Check sheet for the drawn part. Datum: minimum x, y, z corner. Units: mm. A direction names the side the tool comes from. Give positions to 0.01 mm unless a question says otherwise; leave off trailing zeros. Order: outer loops, then holes, each group sorted by start corner. A loop starts at its lowest first (then second) coordinate and runs counter-clockwise, first axis right, second up.
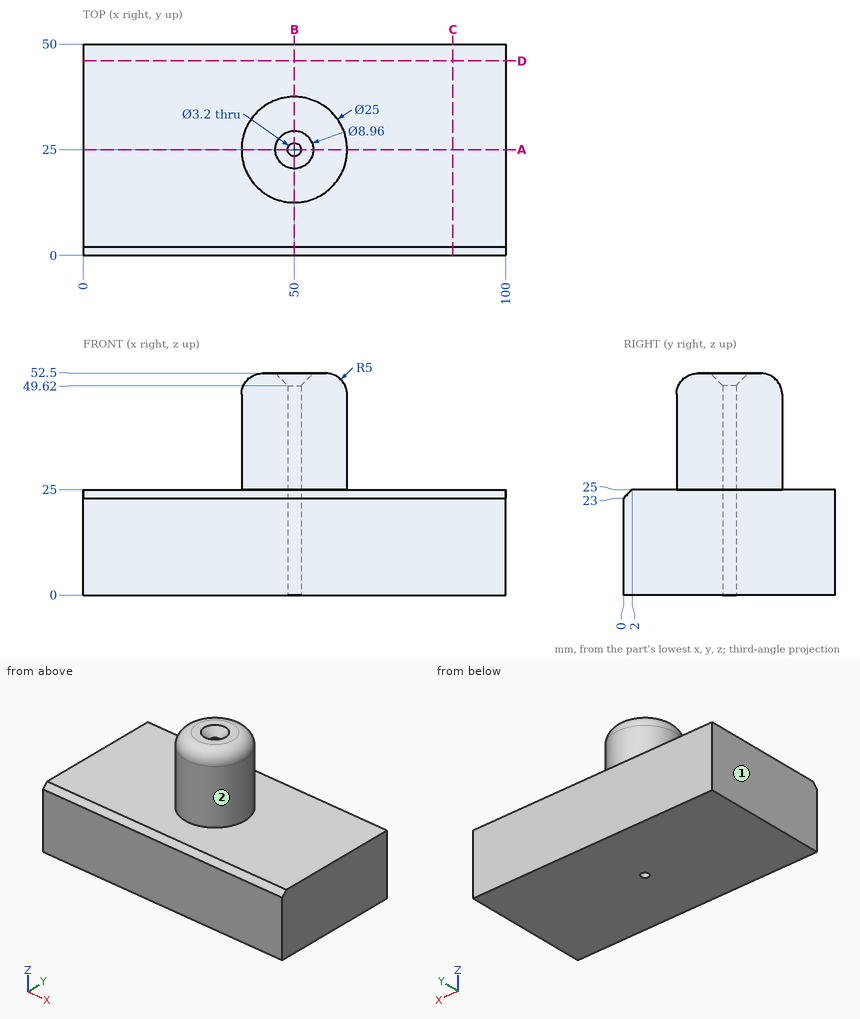
Item 1: Set-up check for the marked faces 1 and 2: record each of +Z, -Z, +X, -X, +Y, -Y from which the full face is reachable in a straight line by a thin tool's end or side.
Reported:
face 1: +Z, -Z, -X, +Y, -Y
face 2: +Z
Item 2: Scan lines: L1, parallel to Y at x = 50, z = 34.5; L2, parallel to X at y = 25, z = 23; L3, parallel to Y at x = 50, z = 14. Record each from-to range of solid material in increasing order.
Reported:
L1: y = 12.5 to 23.4, 26.6 to 37.5
L2: x = 0 to 48.4, 51.6 to 100
L3: y = 0 to 23.4, 26.6 to 50
Item 3: Sectioned sample at B-B (x = 50). Enter the section's corners in (y, z), and give its area (3 significant figures).
Reported:
outline: (0, 0) - (23.4, 0) - (23.4, 49.62) - (20.52, 52.5) - (17.5, 52.5) arc R5 ccw to (12.5, 47.5) - (12.5, 25) - (2, 25) - (0, 23) - close; (26.6, 0) - (50, 0) - (50, 25) - (37.5, 25) - (37.5, 47.5) arc R5 ccw to (32.5, 52.5) - (29.48, 52.5) - (26.6, 49.62) - close
area: 1,750 mm2
Item 4: Sectioned sample at D-D (y = 46). Enter the section's corners in (x, z), and give its area (3 significant figures).
Reported:
outline: (0, 0) - (100, 0) - (100, 25) - (0, 25) - close
area: 2,500 mm2
Item 5: Gauge pin test, flat ends, axial feed: pin 1 (10 mm diameter, centred on y = 35.5, z = 43.5, fed in from +X) (3 decimals); pin 2 (1.9 mm diameter, centred on x = 50, y = 25, fed in from -Z); pin 3 (1 mm diameter, centred on y = 23.5, z = 26.5, fed in from +X). Record the tip position at first contact, or that the pin passes through.
Reported:
pin 1: stops at x = 61.225
pin 2: passes through
pin 3: stops at x = 62.46
Item 6: Sectioned sample at C-C (x = 87.5). Enter the section's corners in (y, z).
Reported:
outline: (0, 0) - (50, 0) - (50, 25) - (2, 25) - (0, 23) - close
Item 7: Sectioned sample at A-A (y = 25). Enter the section's corners in (x, z).
Reported:
outline: (0, 0) - (48.4, 0) - (48.4, 49.62) - (45.52, 52.5) - (42.5, 52.5) arc R5 ccw to (37.5, 47.5) - (37.5, 25) - (0, 25) - close; (51.6, 0) - (100, 0) - (100, 25) - (62.5, 25) - (62.5, 47.5) arc R5 ccw to (57.5, 52.5) - (54.48, 52.5) - (51.6, 49.62) - close
